Here's how the part is built. I have some questions about the finished solid (model axes, mm). A direction names the side the tool comes from. Coordinates: 2 decimals unless noted, no trailing zeros. Write each loop counter-clockwise with the first axis right and the second up, starting at its lowest first coordinate (ties: lowest second). Pieces come first, ordered by that corner, then holes.
```python
from build123d import *

# Parameters (mm, degrees)
SKETCH1_R           = 9.475
BOSS_EXTRUDE1_DEPTH = 13.1
BOSS_EXTRUDE3_DEPTH = 16


with BuildPart() as part:
    # Sketch1 → Boss-Extrude1 (new body)
    with BuildSketch(Plane(origin=(0, 0, 0), x_dir=(1, 0, 0), z_dir=(0, 1, 0))):
        with Locations(Location((0, 0, 0), (0, 0, 270))):
            Circle(SKETCH1_R)
        Polygon((7.361215932, 0), (3.680607966, 6.375), (-3.680607966, 6.375), (-7.361215932, 0), (-3.680607966, -6.375), (3.680607966, -6.375), align=None, mode=Mode.SUBTRACT)
    boss_extrude1 = extrude(amount=BOSS_EXTRUDE1_DEPTH)

    # Sketch2 → Boss-Extrude3 (add)
    with BuildSketch(Plane(origin=(0, 0, 0), x_dir=(1, 0, 0), z_dir=(0, 1, 0))):
        Polygon((-10.2, 6.664466094), (-6.664466094, 10.2), (6.664466094, 10.2), (10.2, 6.664466094), (10.2, -6.664466094), (6.664466094, -10.2), (-6.664466094, -10.2), (-10.2, -6.664466094), align=None)
        Polygon((3.680607966, 6.375), (-3.680607966, 6.375), (-7.361215932, 0), (-3.680607966, -6.375), (3.680607966, -6.375), (7.361215932, 0), align=None, mode=Mode.SUBTRACT)
    extrude(amount=-BOSS_EXTRUDE3_DEPTH)

    # Mirror1: Boss-Extrude1 across plane
    add(boss_extrude1.mirror(Plane.ZX.offset(-8)))


solid = part.part
```
1) We'd pull the mould along X, two halves only. Please class faces 5 (the face through (8.457, -7.888, 8.407)), 6 (the face through (0, -8, 6.375)), 7 (the face through (-8.407, -7.888, 8.457)), 8 (the face through (0, -8, -10.2)): pulls with the +X half, pulls with the -X half, needs draft (parallel to the pull), parting line crosses it, or undercut.
Values follow:
face 5: pulls with the +X half
face 6: undercut
face 7: pulls with the -X half
face 8: needs draft
2) Imagine slicing it at D-D on z = 8.25. Please give me the cut outline in (x, y).
Values follow:
outline: (-8.61, -16) - (-4.66, -16) - (-4.66, -29.1) - (4.66, -29.1) - (4.66, -16) - (8.61, -16) - (8.61, 0) - (4.66, 0) - (4.66, 13.1) - (-4.66, 13.1) - (-4.66, 0) - (-8.61, 0) - close
3) Imagine slicing it at B-B on y = -18.5. Please give me the cut outline in (x, z) (3 decimals).
Values follow:
outline: circle Ø18.95 at (0, 0); hole (-7.361, 0) - (-3.681, -6.375) - (3.681, -6.375) - (7.361, 0) - (3.681, 6.375) - (-3.681, 6.375) - close
4) Imagine slicing it at A-A on x = 0. Please give me the cut outline in (y, z) (3 decimals), then the cut area to 3 significant figures.
Values follow:
outline: (-29.1, -9.475) - (-16, -9.475) - (-16, -10.2) - (0, -10.2) - (0, -9.475) - (13.1, -9.475) - (13.1, -6.375) - (-29.1, -6.375) - close; (-29.1, 6.375) - (13.1, 6.375) - (13.1, 9.475) - (0, 9.475) - (0, 10.2) - (-16, 10.2) - (-16, 9.475) - (-29.1, 9.475) - close
area: 285 mm2
5) Will this pin go through, and if not, where does the flat tip stop? pin 1 (1.5 mm diameter, centred on x = 7.5, y = 6.5, fed in from -Z).
Values follow:
pin 1: stops at z = -6.65
6) On a 3-axis mill with a long thin cutter (end or side, diameter ignored), from which of +Z, -Z, +X, -X, +Y, -Y can I reach the whole of each face in a straight line? I mean faces 1 (the face through (-9.25, -22.46, -2.05)), 2 (the face through (10.2, -8, 0)), 3 (the face through (0, -8, -6.375)), 4 (the face through (8, 0, -6)). Say none if no direction works.
Values follow:
face 1: -Y
face 2: +Z, -Z, +X, +Y, -Y
face 3: +Y, -Y
face 4: +Y
7) I need wall thicknesses on probe 1 along Z at (x, y) = (1, -8.5) (3 decimals); probe 2 along Y at (x, z) = (-8.5, 5.5); probe 3 along X at (y, z) = (3.5, 5.25). Which ranges of each line are inside material? Lowest first, please.
Values follow:
probe 1: z = -10.2 to -6.375, 6.375 to 10.2
probe 2: y = -16 to 0
probe 3: x = -7.89 to -4.33, 4.33 to 7.89
8) Imagine slicing it at C-C on z = 5. Please give me the cut outline in (x, y), then the cut area to 3 significant figures.
Values follow:
outline: (-10.2, -16) - (-8.05, -16) - (-8.05, -29.1) - (-4.47, -29.1) - (-4.47, 13.1) - (-8.05, 13.1) - (-8.05, 0) - (-10.2, 0) - close; (4.47, -29.1) - (8.05, -29.1) - (8.05, -16) - (10.2, -16) - (10.2, 0) - (8.05, 0) - (8.05, 13.1) - (4.47, 13.1) - close
area: 370 mm2
